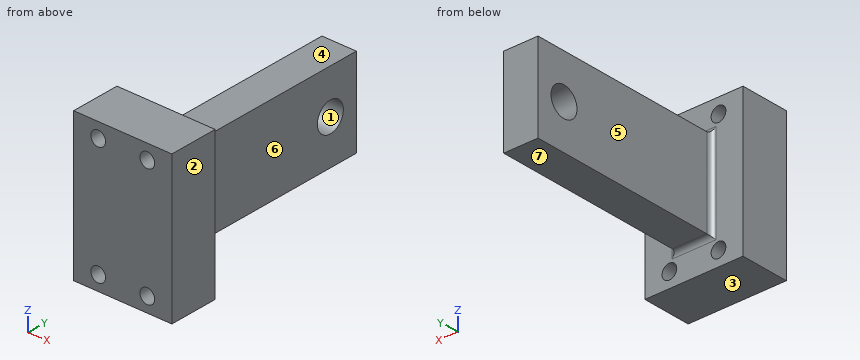
```python
from build123d import *

# Parameters (mm, degrees)
SKETCH1_R           = 1.5
BOSS_EXTRUDE1_DEPTH = 10
SKETCH2_W           = 7
SKETCH2_H           = 18
BOSS_EXTRUDE2_DEPTH = 40
SKETCH3_R           = 3
CUT_EXTRUDE1_DEPTH  = 40
FILLET1_R           = 1


with BuildPart() as part:
    # Sketch1 → Boss-Extrude1 (new body)
    with BuildSketch(Plane(origin=(0, 0, 0), x_dir=(1, 0, 0), z_dir=(0, 1, 0))):
        Polygon((0, 30), (0, 0), (10, 0), (20, 0), (20, 30), align=None)
        with Locations(Location((5, 3, 0), (0, 0, 270))):
            Circle(SKETCH1_R, mode=Mode.SUBTRACT)
        with Locations(Location((15, 3, 0), (0, 0, 270))):
            Circle(SKETCH1_R, mode=Mode.SUBTRACT)
        with Locations(Location((5, 27, 0), (0, 0, 270))):
            Circle(SKETCH1_R, mode=Mode.SUBTRACT)
        with Locations(Location((15, 27, 0), (0, 0, 270))):
            Circle(SKETCH1_R, mode=Mode.SUBTRACT)
    extrude(amount=BOSS_EXTRUDE1_DEPTH)

    # Sketch2 → Boss-Extrude2 (add)
    with BuildSketch(Plane(origin=(0, 10, 0), x_dir=(1, 0, 0), z_dir=(0, 1, 0))):
        with Locations((10, 15)):
            Rectangle(SKETCH2_W, SKETCH2_H)
    extrude(amount=BOSS_EXTRUDE2_DEPTH)

    # Sketch3 → Cut-Extrude1 (cut)
    with BuildSketch(Plane(origin=(13.5, 0, 0), x_dir=(0, 0, -1), z_dir=(1, 0, 0))):
        with Locations((15, 44)):
            Circle(SKETCH3_R)
    extrude(amount=-CUT_EXTRUDE1_DEPTH, mode=Mode.SUBTRACT)

    # Fillet1
    fillet1_edges = [part.edges().sort_by_distance(p)[0] for p in [
        (13.5, 10, -15),
        (10, 10, -24),
        (6.5, 10, -15),
        (10, 10, -6),
    ]]
    fillet(fillet1_edges, radius=FILLET1_R)


solid = part.part
```
Input: part model. Units: mm. Frame: model coordinates. Face numbers are marked on the shaded views. A direction names the side the tool comes from. Coordinates: 2 decimals unless noted, no trailing zeros. Write each loop counter-clockwise with the first axis right and the second up, starting at its lowest first coordinate (ties: lowest second). Pieces come first, ordered by that corner, then holes. Notation, with made-up numbers: (8.25, 59.25) - (60.25, 59.25) arc R8 ccw to (60.25, 74.25) - close; hole circle Ø4 at (76.5, 77.5). An arc over 180 degrees is marked (long way). Put each result on its own line as item: value. Start each with the question number.
1) Cut plane C-C (z = -27). Return the cut outline in (x, y), plus the area to 3 significant figures.
2) Contact query for flat-ended pins moving along their axis: pin 1 (5 mm diameter, centred on y = 44, z = -15, fed in from -X); pin 2 (8 mm diameter, centred on x = 13.5, y = 36, fed in from +Z); pin 3 (3.5 mm diameter, centred on x = 11.5, y = 38.5, fed in from -Z); pin 4 (4 mm diameter, centred on y = 15, z = -21, fed in from +X). Output: stop coordinate, or through.
3) Mould query, pull axis Z, two halves, no side actions, for the marked faces 1, 2, 3 and 4. Classes: pulls with the +Z half, pulls with the -Z half, needs draft (parallel to the pull), parting line crosses it, or undercut.
4) Ray query, L1, parallel to X at y = 7.75, z = -3; L2, parallel to Y at x = 8.75, z = -15; L3, parallel to Y at x = 15, z = -15.25. Return the intervals inside material, ascending.
5) Cut plane D-D (x = 12.5). Return the cut outline in (y, z).
6) Cut plane A-A (y = 4.5). Return the cut outline in (x, z).
7) Cut plane B-B (x = 5). Return the cut outline in (y, z), plus the area to 3 significant figures.
8) Reachability of the marked faces 5, 6 and 7 from +Z, -Z, +X, -X, +Y, -Y: full face, straight path, thin tool, end or side. Return the list, or none.
Resolved:
1. outline: (0, 0) - (3.5, 0) - (3.5, 10) - (0, 10) - close; (6.5, 0) - (13.5, 0) - (13.5, 10) - (6.5, 10) - close; (16.5, 0) - (20, 0) - (20, 10) - (16.5, 10) - close
1. area: 140 mm2
2. pin 1: passes through
2. pin 2: stops at z = -6
2. pin 3: stops at z = -24
2. pin 4: stops at x = 13.5
3. face 1: undercut
3. face 2: needs draft
3. face 3: pulls with the -Z half
3. face 4: pulls with the +Z half
4. L1: x = 0 to 3.5, 6.5 to 13.5, 16.5 to 20
4. L2: y = 0 to 41, 47 to 50
4. L3: y = 0 to 10
5. outline: (0, -30) - (10, -30) - (10, -25) arc R1 cw to (11, -24) - (50, -24) - (50, -6) - (11, -6) arc R1 cw to (10, -5) - (10, 0) - (0, 0) - close; hole circle Ø6 at (44, -15)
6. outline: (0, -30) - (20, -30) - (20, 0) - (0, 0) - close; hole circle Ø3 at (5, -27); hole circle Ø3 at (5, -3); hole circle Ø3 at (15, -27); hole circle Ø3 at (15, -3)
7. outline: (0, -30) - (10, -30) - (10, -28.5) - (0, -28.5) - close; (0, -25.5) - (10, -25.5) - (10, -4.5) - (0, -4.5) - close; (0, -1.5) - (10, -1.5) - (10, 0) - (0, 0) - close
7. area: 240 mm2
8. face 5: +Z, -Z, -X, +Y
8. face 6: +Z, -Z, +X, +Y
8. face 7: -Z, +X, -X, +Y
